from build123d import *

# Parameters (mm, degrees)
BOSS_EXTRU_1_DEPTH = 21
CONG_1_R           = 8
CONG_2_R           = 20
CONG_3_R           = 10


with BuildPart() as part:
    # Esquisse2 → Boss.-Extru.1 (new body)
    with BuildSketch(Plane.XY):
        with BuildLine():
            Line((0, 0), (93.951859629, 0))
            ThreePointArc((93.951859629, 0), (121.451859629, 27.5), (93.951859629, 55))
            Line((93.951859629, 55), (93.951859629, 75))
            ThreePointArc((93.951859629, 75), (141.451859629, 27.5), (93.951859629, -20))
            Line((93.951859629, -20), (-6.305975778, -20))
            Line((-6.305975778, -20), (-90.019669098, 38.616959114))
            Line((-90.019669098, 38.616959114), (-78.548140371, 55))
            Line((-78.548140371, 55), (0, 0))
        make_face()
    extrude(amount=BOSS_EXTRU_1_DEPTH)

    # Congé1
    cong_1_edges = [part.edges().sort_by_distance(p)[0] for p in [
        (93.951859629, 55, 10.5),
        (93.951859629, 75, 10.5),
        (-90.019669098, 38.616959114, 10.5),
        (-78.548140371, 55, 10.5),
    ]]
    fillet(cong_1_edges, radius=CONG_1_R)

    # Congé2
    cong_2_edges = [part.edges().sort_by_distance(p)[0] for p in [
        (-6.305975778, -20, 10.5),
    ]]
    fillet(cong_2_edges, radius=CONG_2_R)

    # Congé3
    cong_3_edges = [part.edges().sort_by_distance(p)[0] for p in [
        (0, 0, 10.5),
    ]]
    fillet(cong_3_edges, radius=CONG_3_R)


solid = part.part
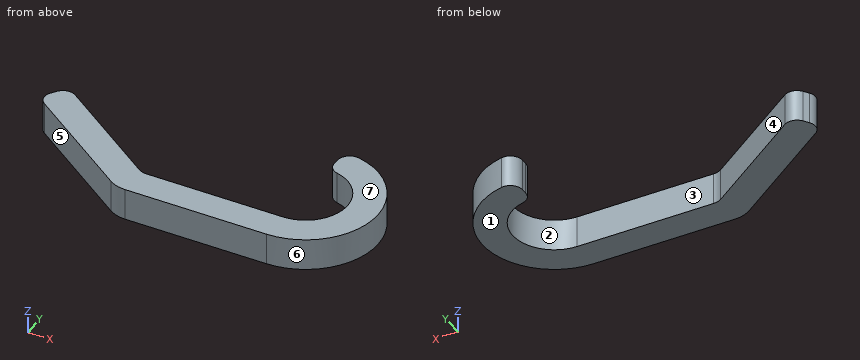
Verification items for the finished model (mm, model axes). Face numbers are marked on the shaded views. A direction names the side the tool comes from. Give positions to 0.01 mm unless a question says otherwise; leave off trailing zeros. Write each loop counter-clockwise with the first axis right and the second up, starting at its lowest first coordinate (ties: lowest second). Pieces come first, ordered by that corner, then holes. Notation, with made-up numbers: M -9,61.5 L 48,61.5 A23 cw 48,73.5 Z; hole C -8.5,66.5 d10. An arc over 180 degrees is marked long. Put each result on its own line as item: value. Start each with the question number.
1. Section check C-C (x = 49). Record the cut outline in (y, z).
2. Set-up check for the marked faces 1, 2 and 3: record each of +Z, -Z, +X, -X, +Y, -Y from which the full face is reachable in a straight line by a thin tool's end or side.
3. Section check D-D (y = 21.5). Record the cut outline in (x, z), and give its area (3 significant figures).
4. Section check A-A (y = 4). Record the cut outline in (x, z), and give its area (3 significant figures).
5. Section check B-B (z = 4.5). Record the cut outline in (x, y).
6. Go/stop test with flat-tipped pins: pin 1 Ø4.5 at (y, z) = (64.5, 13.5) entering from -X; pin 2 Ø10 at (y, z) = (53.5, 9) entering from -X; pin 3 Ø10.5 at (x, z) = (41.5, 12) entering from +Y. Record where each tip stops, or that it passes through.
7. Scan lines: line 1 along Y through (x, z) = (5, 4.5); line 2 along X through (y, z) = (23, 12.75); line 3 along X through (y, z) = (11.5, 7.5). Record each from-to range of solid material in increasing order. Write a range as [from, to].
8. Draft check along X on the marked faces 4, 5, 6 and 7. Enter one of: +X half, -X half, draft (parallel to the pull), parting line (faces both ways), or undercut.
Answer list:
1. outline: M -20,0 L 0,0 L 0,21 L -20,21 Z
2. face 1: -Z, +X, -X, +Y, -Y
2. face 2: +Z, -Z
2. face 3: +Z, -Z, +Y
3. outline: M -65.57,0 L -30.71,0 L -30.71,21 L -65.57,21 Z; M 120.79,0 L 141.07,0 L 141.07,21 L 120.79,21 Z
3. area: 1,160 mm2
4. outline: M -40.58,0 L -5.71,0 L -5.71,21 L -40.58,21 Z; M 108.23,0 L 135.23,0 L 135.23,21 L 108.23,21 Z
4. area: 1,300 mm2
5. outline: M -85.43,45.17 A8 ccw -83.47,34.03 L -11.47,-16.38 A20 ccw 0,-20 L 93.95,-20 A47.5 ccw 103.57,74.02 A8 ccw 93.95,66.18 L 93.95,62.09 A8 ccw 100.15,54.29 A27.5 cw 93.95,0 L 3.15,0 A10 cw -2.58,1.81 L -71.99,50.41 A8 ccw -83.14,48.45 Z
6. pin 1: x = 93.95
6. pin 2: x = -83.1
6. pin 3: y = 0
7. line 1: [-20, 0]
7. line 2: [-67.72, -32.85], [121.08, 141.24]
7. line 3: [-51.29, -16.42], [116.32, 138.68]
8. face 4: undercut
8. face 5: -X half
8. face 6: +X half
8. face 7: draft
